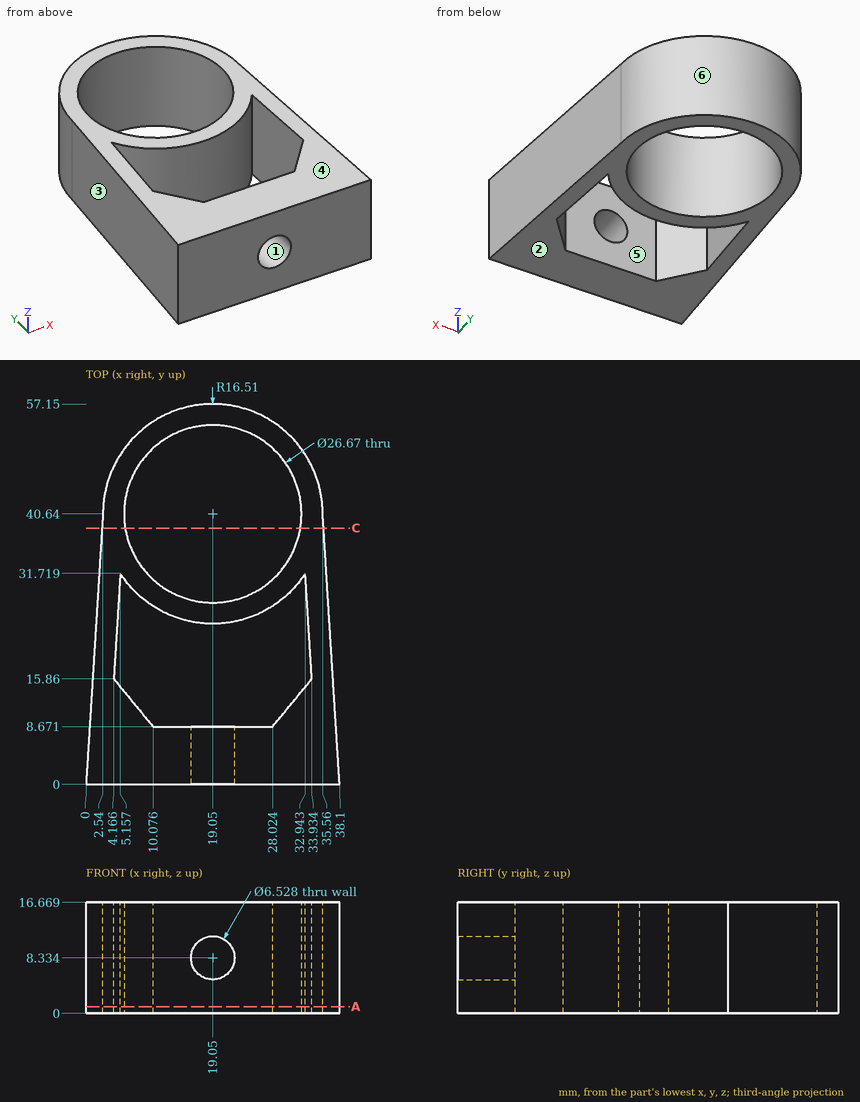
Job drawing, mm, ordinate dimensions from the low corner. One solid piece. A direction names the side the tool comes from. Coordinates: 2 decimals unless noted, no trailing zeros. Order: outer loops, then holes, each group sorted by start corner. A loop starts at its lowest first (then second) coordinate and runs counter-clockwise, first axis right, second up. Notation, with made-up numbers: (-1.75, -20.75) -> (34.25, -20.75) arc R24 cw to (34.25, 4.25) -> close; hole circle Ø3 at (53, -1.5). An arc over 180 degrees is marked (long way). Return JSON: item names as keys, results as strings. Group by question number.
Item 1: Pull direction Z, two halves, no side cores. Call the marked faces 1, 2, 3 and 4: pulls with the +Z half, pulls with the -Z half, needs draft (parallel to the pull), parting line crosses it, or undercut.
Item 2: Saw through at C-C on y = 38.5. Write the cut outline in (x, z), then the cut area to 3 significant figures.
Item 3: Saw through at A-A on z = 1. State how many separate pieces and enclosed holes the cut face has.
Item 4: Tool access for the marked faces 5 and 6: list every direction of +Z, -Z, +X, -X, +Y, -Y with a clear straight run to the whole face (end or side of a thin tool).
Item 5: Wall check: line 1 along Y through (x, z) = (19.5, 13); line 2 along Z through (x, y) = (19.05, 3.5); line 3 along Y through (x, z) = (14.5, 3.5) (1 decimal). Give the ranges that are in metal, low to high. Write a range as [from, to].
Item 6: Flat gauge pins, fed straight in: P1, Ø3, axis at y = 14.5, z = 7, coming from the -X side; P2, Ø5, axis at y = 48.5, z = 8.5, coming from the -X side (1 decimal). Where does each tip first touch, or does it go through?
Values found:
{
 "1": {"face 1": "undercut", "face 2": "pulls with the -Z half", "face 3": "needs draft", "face 4": "pulls with the +Z half"},
 "2": {"outline": "(2.41, 0) -> (5.89, 0) -> (5.89, 16.67) -> (2.41, 16.67) -> close; (32.21, 0) -> (35.69, 0) -> (35.69, 16.67) -> (32.21, 16.67) -> close", "area": "116 mm2"},
 "3": {"separate pieces": "1", "enclosed holes": "2"},
 "4": {"face 5": "+Z, -Z", "face 6": "+Z, -Z, +Y"},
 "5": {"line 1": "y = [0, 8.67], [24.14, 27.31], [53.97, 57.14]", "line 2": "z = [0, 5.07], [11.6, 16.67]", "line 3": "y = [0, 8.7], [24.8, 28.1], [53.2, 56.5]"},
 "6": {"P1": "stops at x = 0.81", "P2": "stops at x = 3.4"}
}
